Geometry check sheet. Reference: drawing and pictorial views, mm from the part's lowest x, y, z. Round coordinates to 2 decimals unless told otherwise and drop trailing zeros. Order: outer loops, then holes, each group sorted by start corner. A loop starts at its lowest first (then second) coordinate and runs counter-clockwise, first axis right, second up.
(1) Sectioned sample at A-A (x = 5). Record the boundary of the cut face in (y, z).
(2) Go/stop test with flat-tipped pins: pin 1 (1.9 mm diameter, centred on y = 245, z = 5, fed in from -X); pin 2 (6 mm diameter, centred on y = 70.5, z = 4, fed in from -X). Record where each tip stops, or that it passes through.
(3) Material ranges on line 1 along Y through (x, z) = (5, 7.5); line 2 along Z through (x, y) = (7.5, 5); line 3 along Y through (x, z) = (2.5, 5), recorded low to high.
(4) Sectioned sample at B-B (z = 5). Record the boundary of the cut face in (x, y).
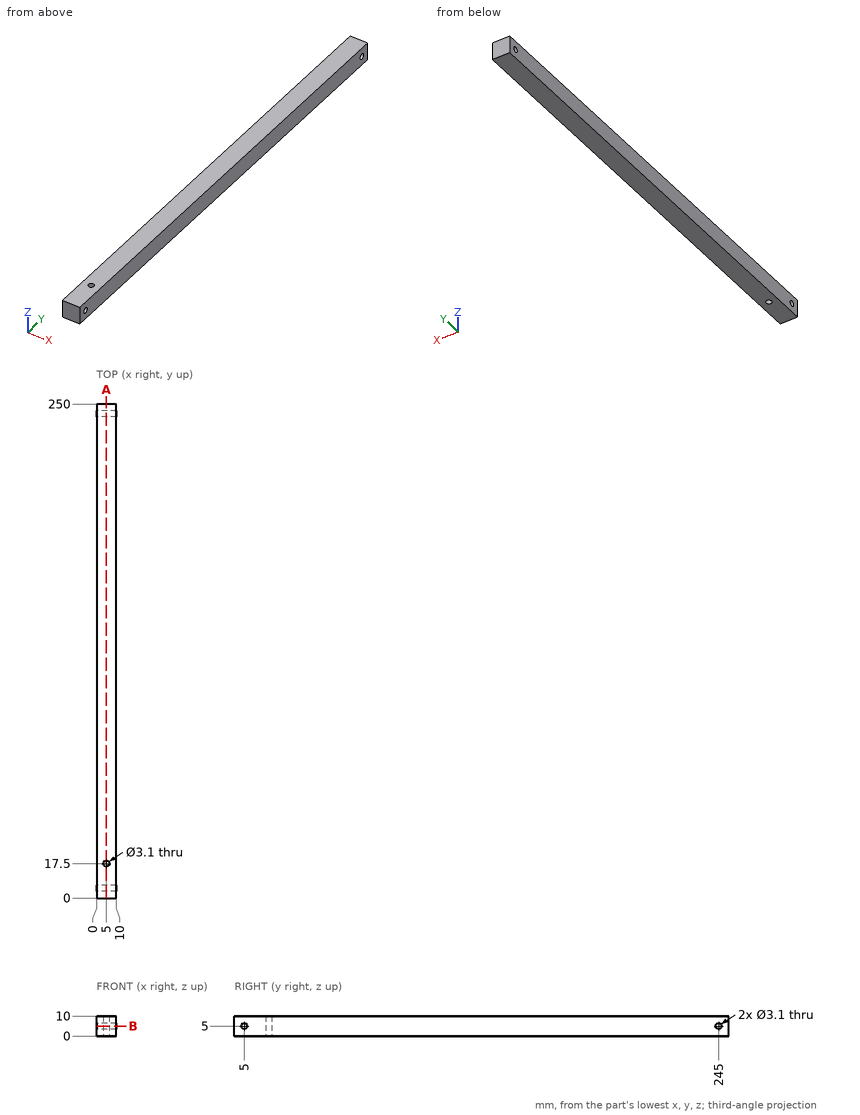
Answer below:
1. outline: (0, 0) - (15.95, 0) - (15.95, 10) - (0, 10) - close; (19.05, 0) - (250, 0) - (250, 10) - (19.05, 10) - close; hole circle Ø3.1 at (5, 5); hole circle Ø3.1 at (245, 5)
2. pin 1: passes through
2. pin 2: stops at x = 0
3. line 1: y = 0 to 15.95, 19.05 to 250
3. line 2: z = 0 to 3.45, 6.55 to 10
3. line 3: y = 0 to 3.45, 6.55 to 243.45, 246.55 to 250
4. outline: (0, 0) - (10, 0) - (10, 3.45) - (0, 3.45) - close; (0, 6.55) - (10, 6.55) - (10, 243.45) - (0, 243.45) - close; (0, 246.55) - (10, 246.55) - (10, 250) - (0, 250) - close; hole circle Ø3.1 at (5, 17.5)
